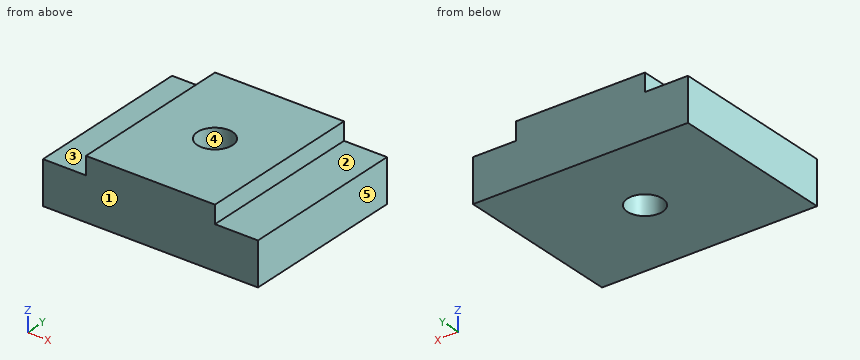
from build123d import *

# Parameters (mm, degrees)
BOSS_EXTRUDE1_DEPTH = 20
SKETCH2_R           = 2.0828
CUT_EXTRUDE1_DEPTH  = 25.791990194


with BuildPart() as part:
    # Sketch1 → Boss-Extrude1 (new body)
    with BuildSketch(Plane(origin=(0, 0, 0), x_dir=(1, 0, 0), z_dir=(0, 1, 0))):
        Polygon((7.65, 0), (-7.65, 0), (-7.65, 2.116666667), (-12.75, 2.116666667), (-12.75, 7.216666667), (12.75, 7.216666667), (12.75, 2.116666667), (7.65, 2.116666667), align=None)
    extrude(amount=BOSS_EXTRUDE1_DEPTH)

    # Sketch2 → Cut-Extrude1 (cut, through all)
    with BuildSketch(Plane(origin=(0, 0, -7.216666667), x_dir=(-1, 0, 0), z_dir=(0, 0, -1))):
        with Locations((0, 10)):
            Circle(SKETCH2_R)
    extrude(amount=-CUT_EXTRUDE1_DEPTH, mode=Mode.SUBTRACT)


solid = part.part
Design review of the part built by this model. Coordinates are the model's own, in mm. Face numbers are marked on the shaded views. A direction names the side the tool comes from. Round coordinates to 2 decimals unless told otherwise and drop trailing zeros. Write each loop counter-clockwise with the first axis right and the second up, starting at its lowest first coordinate (ties: lowest second). Pieces come first, ordered by that corner, then holes. Notation, with made-up numbers: M -3,52.5 L 24,52.5 A15 ccw 24,56.5 Z; hole C 82,-10 d2. An arc over 180 degrees is marked long. One line per item, written item: value. Start each with the question number.
1. Take a section at B-B on y = 10. State the section outline as (x, z) points.
2. For the marked faces 1 and 2, list the 3-axis set-ups (+Z, -Z, +X, -X, +Y, -Y) from which the entire face can be reached by the end or side of a thin tool; tool diameter is ignored.
3. To check wall thickness, follow probe 1 along Y at (x, z) = (0, -3.75); probe 2 along X at (y, z) = (1.25, -2); probe 3 along Y at (x, z) = (-1.5, -2.25). State the ranges of each line that lie inside material, in increasing order. Write a range as from..to.
4. Take a section at A-A on x = 0. State the section outline as (y, z) points, then the cut area to 3 significant figures.
5. Take a section at C-C on z = -4.75. State the section outline as (x, y) points.
6. Take a section at D-D on y = 18.75. State the section outline as (x, z) points.
7. Clearance check with flat-ended pins moving along their axes: P1, Ø3.5, axis at x = 0, y = 10, coming from the -Z side; P2, Ø1.7, axis at y = 8.5, z = -1, coming from the -X side; P3, Ø5.5, axis at x = 11, y = 10.5, coming from the +Z side; P4, Ø0.6, axis at y = 10, z = -1, coming from the +X side. State where each tip first meets the part, or that it passes through.
8. Draft analysis for pull direction X (two halves, no side actions). For the marked faces 3, 4 and 5, state which applies: pulls with the +X half, pulls with the -X half, needs draft (parallel to the pull), parting line crosses it, or undercut.
Computed:
1. outline: M -12.75,-7.22 L -2.08,-7.22 L -2.08,0 L -7.65,0 L -7.65,-2.12 L -12.75,-2.12 Z; M 2.08,-7.22 L 12.75,-7.22 L 12.75,-2.12 L 7.65,-2.12 L 7.65,0 L 2.08,0 Z
2. face 1: +Z, -Z, +X, -X, -Y
2. face 2: +Z, +X, +Y, -Y
3. probe 1: y = 0..7.92, 12.08..20
3. probe 2: x = -7.65..7.65
3. probe 3: y = 0..8.55, 11.45..20
4. outline: M 0,-7.22 L 7.92,-7.22 L 7.92,0 L 0,0 Z; M 12.08,-7.22 L 20,-7.22 L 20,0 L 12.08,0 Z
4. area: 114 mm²
5. outline: M -12.75,0 L 12.75,0 L 12.75,20 L -12.75,20 Z; hole C 0,10 d4.17
6. outline: M -12.75,-7.22 L 12.75,-7.22 L 12.75,-2.12 L 7.65,-2.12 L 7.65,0 L -7.65,0 L -7.65,-2.12 L -12.75,-2.12 Z
7. P1: passes through
7. P2: stops at x = -7.65
7. P3: stops at z = -2.12
7. P4: stops at x = 7.65
8. face 3: needs draft
8. face 4: undercut
8. face 5: pulls with the +X half
